```python
from build123d import *

# Parameters (mm, degrees)
F0_W     = 228.6
F0_H     = 450.85
F1_DEPTH = 546.1
F2_T     = -2.54


with BuildPart() as f1:
    # F0 (on Front) → F1 (new body)
    with BuildSketch(Plane.XZ):
        Rectangle(F0_W, F0_H)
    extrude(amount=-F1_DEPTH)

    # F2
    f2_openings = [f1.faces().sort_by_distance(p)[0] for p in [
        (114.3, 273.05, 0),
    ]]
    offset(amount=F2_T, openings=f2_openings)


solid = f1.part
```
CAD build for the part. Positions are in the model's coordinates, mm. A direction names the side the tool comes from. Coordinates: 2 decimals unless noted, no trailing zeros. Order: outer loops, then holes, each group sorted by start corner. A loop starts at its lowest first (then second) coordinate and runs counter-clockwise, first axis right, second up. Notation, with made-up numbers: M 42,83 L 75,83 A16 cw 75,87 Z; hole C 72,-26.5 d10. An arc over 180 degrees is marked long. Write each question's results on one line, items separated by ' | '. Start each with the question number.
Q1. Cut at B-B (z = 23). List the corners of the cut face in (x, y).
Q2. Drill centre lines: probe 1 along Z at (x, y) = (-92, 295) (3 decimals); probe 2 along Y at (x, z) = (-67.5, 103); probe 3 along X at (y, z) = (108, -120.5). Where is each one in solid material? Low to high. Write a range as from..to.
Q3. Flat gauge pin, fed straight in: P1, Ø3, axis at y = 64, z = -17.5, coming from the +X side. Where does the tip first touch, or does it go through?
Q4. Cut at A-A (x = 1). List the corners of the cut face in (y, z) (3 decimals), then the cut area to 3 significant figures.
Q5. Pull direction Z, two halves, no side cores. Call faces 3 (the flat face through (-2, 269, -225.425)), 4 (the flat face through (0, 543.56, 3)), 5 (the flat face through (-114.3, 269, -3)): +Z half, -Z half, draft (parallel to the pull), parting line (faces both ways), or undercut.
Q6. Cut at C-C (y = 176). List the corners of the cut face in (x, z) (3 decimals), then the cut area to 3 significant figures.
Q7. Which spindle directions (+Z, -Z, +X, -X, +Y, -Y) get a long thin tool onto all of the face, cutting with end or side? Do faces 1 (the flat face through (-2, 269, 225.425)), 2 (the flat face through (0, 269, 222.885)). Say none if no direction does.
Found:
1) outline: M -114.3,0 L 114.3,0 L 114.3,2.54 L -111.76,2.54 L -111.76,543.56 L 114.3,543.56 L 114.3,546.1 L -114.3,546.1 Z
2) probe 1: -225.425..-222.885, 222.885..225.425 | probe 2: 0..2.54, 543.56..546.1 | probe 3: -114.3..-111.76
3) P1: x = -111.76
4) outline: M 0,-225.425 L 546.1,-225.425 L 546.1,225.425 L 0,225.425 Z; hole M 2.54,-222.885 L 543.56,-222.885 L 543.56,222.885 L 2.54,222.885 Z | area: 5,040 mm²
5) face 3: -Z half | face 4: undercut | face 5: draft
6) outline: M -114.3,-225.425 L 114.3,-225.425 L 114.3,-222.885 L -111.76,-222.885 L -111.76,222.885 L 114.3,222.885 L 114.3,225.425 L -114.3,225.425 Z | area: 2,290 mm²
7) face 1: +Z, +X, -X, +Y, -Y | face 2: +X
